```python
from build123d import *

# Parameters (mm, degrees)
CROQUIS1_W              = 142
CROQUIS1_H              = 20.7
CROQUIS1_H_2            = 2.15
SALIENTE_EXTRUIR1_DEPTH = 15
CROQUIS2_W              = 21
CROQUIS2_H              = 13
CORTAR_EXTRUIR1_DEPTH   = 230
SALIENTE_EXTRUIR4_DEPTH = 142
CROQUIS12_W             = 16.7
CROQUIS12_H             = 9.7
CORTAR_EXTRUIR2_DEPTH   = 10


with BuildPart() as part:
    # Croquis1 → Saliente-Extruir1 (new body)
    with BuildSketch(Plane(origin=(0, 0, 0), x_dir=(1, 0, 0), z_dir=(0, 1, 0))):
        Rectangle(CROQUIS1_W, CROQUIS1_H)
        with Locations((0, 11.425)):
            Rectangle(CROQUIS1_W, CROQUIS1_H_2)
        with Locations((0, -11.425)):
            Rectangle(CROQUIS1_W, CROQUIS1_H_2)
    extrude(amount=SALIENTE_EXTRUIR1_DEPTH)

    # Croquis2 → Cortar-Extruir1 (cut)
    with BuildSketch(Plane.ZY.offset(71)):
        with Locations((0, 6.5)):
            Rectangle(CROQUIS2_W, CROQUIS2_H)
    extrude(amount=-CORTAR_EXTRUIR1_DEPTH, mode=Mode.SUBTRACT)

    # Croquis11 → Saliente-Extruir4 (add)
    with BuildSketch(Plane.ZY.offset(71)):
        Polygon((-10.5, 1.35), (-10.5, 2.55), (-10, 2.55), align=None)
        Polygon((10, 2.55), (10.5, 1.35), (10.5, 2.55), align=None)
    extrude(amount=-SALIENTE_EXTRUIR4_DEPTH)

    # Croquis12 → Cortar-Extruir2 (cut)
    with BuildSketch(Plane.XY.offset(12.5)):
        with Locations((0, 7.85)):
            Rectangle(CROQUIS12_W, CROQUIS12_H)
    extrude(amount=-CORTAR_EXTRUIR2_DEPTH, mode=Mode.SUBTRACT)


solid = part.part
```
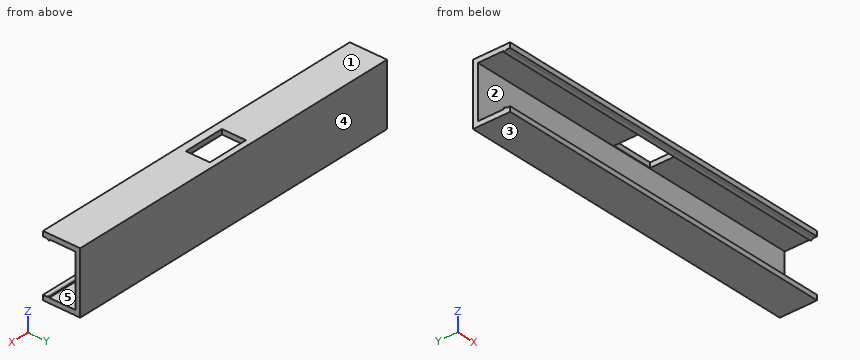
Build history of the part. All positions in model axes, mm. Face numbers are marked on the shaded views. A direction names the side the tool comes from. Round coordinates to 2 decimals unless told otherwise and drop trailing zeros. Write each loop counter-clockwise with the first axis right and the second up, starting at its lowest first coordinate (ties: lowest second). Pieces come first, ordered by that corner, then holes. Notation, with made-up numbers: (79, 7.5) - (126, 7.5) arc R17 cw to (126, 40.5) - close; hole circle Ø7 at (-37, -19). An arc over 180 degrees is marked (long way). Write each question's results on one line, items separated by ' | '. Start each with the question number.
Item 1: Saw through at C-C (x = -46). Write the cut outline in (y, z).
Item 2: Drop a flat-ended pin along its axis: P1, Ø5, axis at x = -14, z = -4, coming from the -Y side. Give the stop position or say it passes through.
Item 3: Mould opens along Z. For the marked faces 1, 2 and 3 say: pulls with the +Z half, pulls with the -Z half, needs draft (parallel to the pull), parting line crosses it, or undercut.
Item 4: Wall check: L1, parallel to Z at x = -39.5, y = 3; L2, parallel to Z at x = 3.5, y = 2.5; L3, parallel to X at y = 9, z = 10.75. Give the ranges that are in metal, low to high. Write a range as [from, to].
Item 5: Saw through at D-D (z = 1.25). Write the cut outline in (x, y).
Item 6: Which spindle directions (+Z, -Z, +X, -X, +Y, -Y) get a long thin tool onto all of the face, cutting with end or side? Do the marked faces 4 and 5. Say none if no direction does.
Item 7: Saw through at B-B (x = 0). Write the cut outline in (y, z), and give its area (3 significant figures).
Item 8: Saw through at A-A (y = 9.25). Write the cut outline in (x, z), and give its area (3 significant figures).
Results are:
1) outline: (0, -12.5) - (15, -12.5) - (15, 12.5) - (0, 12.5) - (0, 10.5) - (1.35, 10.5) - (2.55, 10) - (2.55, 10.5) - (13, 10.5) - (13, -10.5) - (2.55, -10.5) - (2.55, -10) - (1.35, -10.5) - (0, -10.5) - close
2) P1: stops at y = 13
3) face 1: pulls with the +Z half | face 2: undercut | face 3: pulls with the -Z half
4) L1: z = [-12.5, -10.5], [10.5, 12.5] | L2: z = [-12.5, -10.02], [10.02, 12.5] | L3: x = [-71, -8.35], [8.35, 71]
5) outline: (-71, 13) - (71, 13) - (71, 15) - (-71, 15) - close
6) face 4: +Z, -Z, +X, -X, +Y | face 5: +X, -X
7) outline: (0, -12.5) - (15, -12.5) - (15, 12.5) - (12.7, 12.5) - (12.7, 10.5) - (13, 10.5) - (13, -10.5) - (2.55, -10.5) - (2.55, -10) - (1.35, -10.5) - (0, -10.5) - close; (0, 10.5) - (1.35, 10.5) - (2.55, 10) - (2.55, 10.5) - (3, 10.5) - (3, 12.5) - (0, 12.5) - close | area: 83.2 mm²
8) outline: (-71, -12.5) - (71, -12.5) - (71, -10.5) - (-71, -10.5) - close; (-71, 10.5) - (-8.35, 10.5) - (-8.35, 12.5) - (-71, 12.5) - close; (8.35, 10.5) - (71, 10.5) - (71, 12.5) - (8.35, 12.5) - close | area: 535 mm²
